Autodesk Fusion 360 part; units mm, degrees
sketch "Plate" plane through (0, 0, 0) normal (0, 0, 1) x (1, 0, 0)
  line L0 (-111, 0.4) -> (111, 0.4)
  line L1 (111, 0.4) -> (111, 44.05)
  line L2 (111, 44.05) -> (-111, 44.05)
  line L3 (-111, 44.05) -> (-111, 0.4)
extrude "Plate (1)" add sketch "Plate" along normal blind 4
sketch "Duct walls" plane through (0, 0, 0) normal (0, 0, 1) x (1, 0, 0)
  line L0 (-97.22, 2.1) -> (97.22, 2.1)
  line L1 (97.22, 2.1) -> (97.22, 4.3)
  line L2 (97.22, 4.3) -> (-97.22, 4.3)
  line L3 (-97.22, 4.3) -> (-97.22, 2.1)
  line L4 (-97.22, 40.15) -> (97.22, 40.15)
  line L5 (97.22, 40.15) -> (97.22, 42.35)
  line L6 (97.22, 42.35) -> (-97.22, 42.35)
  line L7 (-97.22, 42.35) -> (-97.22, 40.15)
extrude "Duct walls (1)" add sketch "Duct walls" against normal blind 72
sketch "Openings and holes" plane through (0, 0, 0) normal (0, 0, 1) x (1, 0, 0)
  circle A0 centre (-63.55, 22.225) radius 19.5
  circle A1 centre (-79.55, 6.225) radius 1.8
  circle A2 centre (-79.55, 38.225) radius 1.8
  circle A3 centre (-47.55, 6.225) radius 1.8
  circle A4 centre (-47.55, 38.225) radius 1.8
  circle A5 centre (0, 22.225) radius 19.5
  circle A6 centre (-16, 6.225) radius 1.8
  circle A7 centre (-16, 38.225) radius 1.8
  circle A8 centre (16, 6.225) radius 1.8
  circle A9 centre (16, 38.225) radius 1.8
  circle A10 centre (63.55, 22.225) radius 19.5
  circle A11 centre (47.55, 6.225) radius 1.8
  circle A12 centre (47.55, 38.225) radius 1.8
  circle A13 centre (79.55, 6.225) radius 1.8
  circle A14 centre (79.55, 38.225) radius 1.8
  circle A15 centre (-102.82, 15) radius 1.7
  circle A16 centre (-102.82, 29.45) radius 1.7
  circle A17 centre (102.82, 15) radius 1.7
  circle A18 centre (102.82, 29.45) radius 1.7
extrude "Openings and holes (1)" cut sketch "Openings and holes" along normal blind 4
sketch "Tie slots" plane through (0, 0, 0) normal (0, 0, 1) x (1, 0, 0)
  line L0 (-33.03, 15) -> (-30.53, 15)
  line L1 (-30.53, 15) -> (-30.53, 20)
  line L2 (-30.53, 20) -> (-33.03, 20)
  line L3 (-33.03, 20) -> (-33.03, 15)
  line L4 (-33.03, 24.5) -> (-30.53, 24.5)
  line L5 (-30.53, 24.5) -> (-30.53, 29.5)
  line L6 (-30.53, 29.5) -> (-33.03, 29.5)
  line L7 (-33.03, 29.5) -> (-33.03, 24.5)
  line L8 (30.53, 15) -> (33.03, 15)
  line L9 (33.03, 15) -> (33.03, 20)
  line L10 (33.03, 20) -> (30.53, 20)
  line L11 (30.53, 20) -> (30.53, 15)
  line L12 (30.53, 24.5) -> (33.03, 24.5)
  line L13 (33.03, 24.5) -> (33.03, 29.5)
  line L14 (33.03, 29.5) -> (30.53, 29.5)
  line L15 (30.53, 29.5) -> (30.53, 24.5)
  line L16 (88.19, 15) -> (90.69, 15)
  line L17 (90.69, 15) -> (90.69, 20)
  line L18 (90.69, 20) -> (88.19, 20)
  line L19 (88.19, 20) -> (88.19, 15)
  line L20 (88.19, 24.5) -> (90.69, 24.5)
  line L21 (90.69, 24.5) -> (90.69, 29.5)
  line L22 (90.69, 29.5) -> (88.19, 29.5)
  line L23 (88.19, 29.5) -> (88.19, 24.5)
extrude "Tie slots (1)" cut sketch "Tie slots" along normal blind 4
ref_plane "WorkPlane1" through (0, 0, 4) normal (0, 0, 1) x (1, 0, 0)
sketch "Head counterbores" plane through (0, 0, 4) normal (0, 0, 1) x (1, 0, 0)
  circle A0 centre (-102.82, 15) radius 3.25
  circle A1 centre (-102.82, 29.45) radius 3.25
  circle A2 centre (102.82, 15) radius 3.25
  circle A3 centre (102.82, 29.45) radius 3.25
extrude "Head counterbores (1)" cut sketch "Head counterbores" against normal blind 2
CAD build for the part. Positions are in the model's coordinates, mm. A direction names the side the tool comes from. Coordinates: 2 decimals unless noted, no trailing zeros. Order: outer loops, then holes, each group sorted by start corner. A loop starts at its lowest first (then second) coordinate and runs counter-clockwise, first axis right, second up. Notation, with made-up numbers: (-22.5, -26.5) - (3.5, -26.5) arc R25 ccw to (3.5, 9.5) - close; hole circle Ø8 at (4.25, -35). An arc over 180 degrees is marked (long way). Use a Markdown table: item, result. Add a question column.
(1) Saw through at C-C (x = 40). Give the cut face in (y, z), then the cut area to 3 significant figures.
(2) Pull direction Y, two halves, no side cores. Call faces 4 (the face through (-2, 42, 4)), 5 (the face through (-2, 0.4, 2)), 6 (the face through (105.92, 15.98, 3.01)): +Y half, -Y half, draft (parallel to the pull), parting line (faces both ways), or undercut.
(3) Saw through at D-D (x = -66.5). Give the cut face in (y, z), then the cut area to 3 significant figures.
(4) Drill centre lines: line 1 along Y through (x, z) = (-62, -4); line 2 along Y through (x, z) = (-79.55, 1.7) (3 decimals); line 3 along Y through (x, z) = (47, 1). Where is each one in solid material? Low to high. Write a range as [from, to].
(5) Saw through at A-A (z = -42). Give the cut face in (x, y).
(6) Flat gauge pins, fed straight in: pin 1 (4 mm diameter, centred on y = 39.5, z = -50.5, fed in from -X); pin 2 (2 mm diameter, centred on x = -60.5, z = -9.5, fed in from -Y); pin 3 (10 mm diameter, centred on y = 36, z = -46.5, fed in from +X). Where does each tip first touch, or does it go through?
(7) Saw through at B-B (x = 0). Give the cut face in (y, z) (3 decimals).
(8) Which spindle directions (+Z, -Z, +X, -X, +Y, -Y) get a long thin tool onto all of the face, cutting with end or side? Do faces 1 (the face through (33.03, 27, 2)), 2 (the face through (111, 22, 2)), 3 (the face through (-101, 28, 2)). Say none if no direction does.
Solved:
| question | item | result |
|---|---|---|
| 1 | outline | (0.4, 0) - (2.1, 0) - (2.1, -72) - (4.3, -72) - (4.3, 0) - (40.15, 0) - (40.15, -72) - (42.35, -72) - (42.35, 0) - (44.05, 0) - (44.05, 4) - (0.4, 4) - close |
| 1 | area | 491 mm² |
| 2 | face 4 | draft |
| 2 | face 5 | -Y half |
| 2 | face 6 | undercut |
| 3 | outline | (0.4, 0) - (2.1, 0) - (2.1, -72) - (4.3, -72) - (4.3, 0) - (2.95, 0) - (2.95, 4) - (0.4, 4) - close; (40.15, -72) - (42.35, -72) - (42.35, 0) - (44.05, 0) - (44.05, 4) - (41.5, 4) - (41.5, 0) - (40.15, 0) - close |
| 3 | area | 337 mm² |
| 4 | line 1 | y = [2.1, 4.3], [40.15, 42.35] |
| 4 | line 2 | y = [0.4, 4.425], [8.025, 11.078], [33.372, 36.425], [40.025, 44.05] |
| 4 | line 3 | y = [0.4, 4.51], [7.94, 11.91], [32.54, 36.51], [39.94, 44.05] |
| 5 | outline | (-97.22, 2.1) - (97.22, 2.1) - (97.22, 4.3) - (-97.22, 4.3) - close; (-97.22, 40.15) - (97.22, 40.15) - (97.22, 42.35) - (-97.22, 42.35) - close |
| 6 | pin 1 | stops at x = -97.22 |
| 6 | pin 2 | stops at y = 2.1 |
| 6 | pin 3 | stops at x = 97.22 |
| 7 | outline | (0.4, 0) - (2.1, 0) - (2.1, -72) - (4.3, -72) - (4.3, 0) - (2.725, 0) - (2.725, 4) - (0.4, 4) - close; (40.15, -72) - (42.35, -72) - (42.35, 0) - (44.05, 0) - (44.05, 4) - (41.725, 4) - (41.725, 0) - (40.15, 0) - close |
| 8 | face 1 | +Z, -Z |
| 8 | face 2 | +Z, -Z, +X, +Y, -Y |
| 8 | face 3 | +Z |
